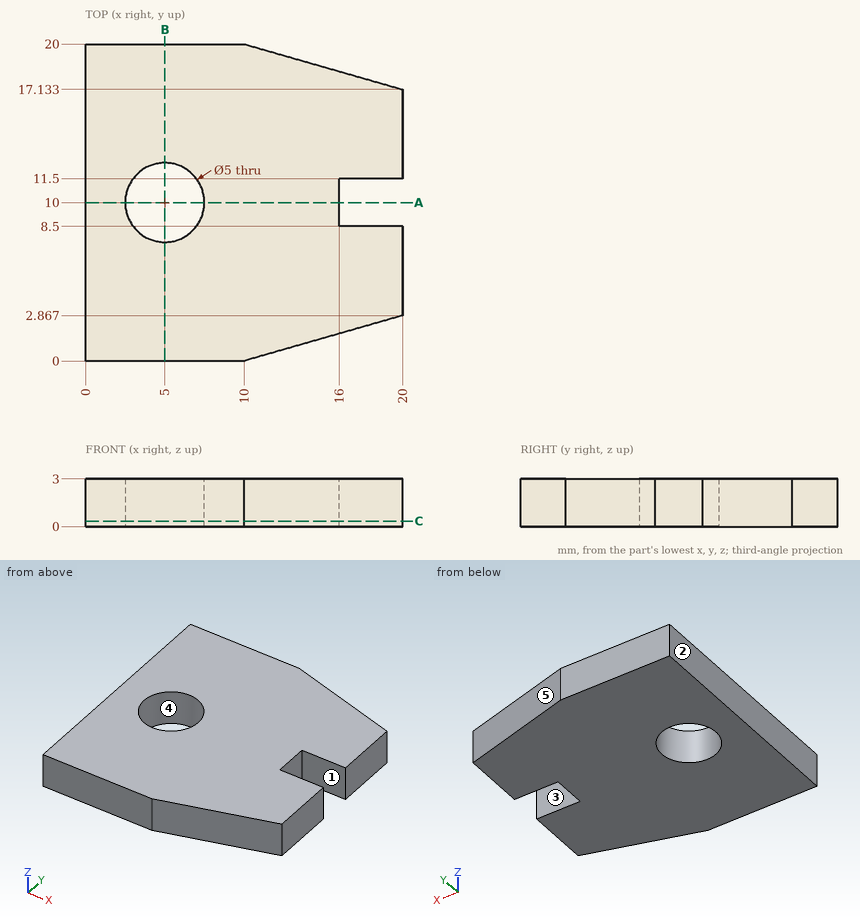
Answer from the drawing. Dimensions are ordinates in mm from the lowest x, y and z of the part. A direction names the side the tool comes from. Coordinates: 2 decimals unless noted, no trailing zeros. Write each loop counter-clockwise with the first axis right and the second up, starting at its lowest first coordinate (ties: lowest second). Pieces come first, ordered by that corner, then holes. Notation, with made-up numbers: (15, 46) - (38, 46) arc R10 cw to (38, 50) - close; hole circle Ø6 at (42.5, 8.25). An arc over 180 degrees is marked (long way). Return JSON: item names as keys, results as strings. Group by question number.
Q1. The part is cut by section A-A on y = 10. Write down the section's boundary in (x, z).
Q2. Which of the six approach directions +Z, -Z, +X, -X, +Y, -Y give full straight-line access (tool end or side, diameter ignored) to the marked faces 1 and 2?
Q3. The part is cut by section B-B on x = 5. Write down the section's boundary in (y, z).
Q4. Find the intervals of material crossed by line 1 along Y through (x, z) = (5, 1.75); line 2 along Y through (x, z) = (18, 2.2) (1 decimal); line 3 along X through (y, z) = (10.5, 2.15), in increasing order. Write a range as [from, to].
Q5. Flat-ended cylindrical pins translate along their axes: pin 1 Ø1 at (y, z) = (13, 2.5) entering from -X; pin 2 Ø0.9 at (x, z) = (17.5, 1) entering from -Y; pin 3 Ø0.9 at (x, z) = (18, 1) entering from +Y (1 decimal). Find the tip coordinate at first contact, or state that the pin passes through.
Q6. The part is cut by section C-C on z = 0.35. Write down the section's boundary in (x, y).
Q7. For a pull along X with two mould halves and no side action, classify the marked faces 3, 4 and 5 as +X half, -X half, draft (parallel to the pull), parting line (faces both ways), or undercut.
Evaluation:
{
 "1": {"outline": "(0, 0) - (2.5, 0) - (2.5, 3) - (0, 3) - close; (7.5, 0) - (16, 0) - (16, 3) - (7.5, 3) - close"},
 "2": {"face 1": "+Z, -Z, +X", "face 2": "+Z, -Z, -X, +Y, -Y"},
 "3": {"outline": "(0, 0) - (7.5, 0) - (7.5, 3) - (0, 3) - close; (12.5, 0) - (20, 0) - (20, 3) - (12.5, 3) - close"},
 "4": {"line 1": "y = [0, 7.5], [12.5, 20]", "line 2": "y = [2.3, 8.5], [11.5, 17.7]", "line 3": "x = [0, 2.55], [7.45, 16]"},
 "5": {"pin 1": "stops at x = 0", "pin 2": "stops at y = 2.02", "pin 3": "stops at y = 17.8"},
 "6": {"outline": "(0, 0) - (10, 0) - (20, 2.87) - (20, 8.5) - (16, 8.5) - (16, 11.5) - (20, 11.5) - (20, 17.13) - (10, 20) - (0, 20) - close; hole circle Ø5 at (5, 10)"},
 "7": {"face 3": "draft", "face 4": "undercut", "face 5": "+X half"}
}
